Work out the finished part from the listing and answer in its coordinate system (mm). A direction names the side the tool comes from. Round coordinates to 2 decimals unless told otherwise and drop trailing zeros. Write each loop counter-clockwise with the first axis right and the second up, starting at its lowest first coordinate (ties: lowest second). Pieces come first, ordered by that corner, then holes.
1. Flat-ended cylindrical pins translate along their axes: pin 1 Ø1.5 at (x, y) = (16, -24.5) entering from +Z; pin 2 Ø6 at (x, z) = (19, 1) entering from -Y; pin 3 Ø3 at (y, z) = (18.5, 6) entering from -X. Find the tip coordinate at first contact, or state that the pin passes through.
2. Find section B-B (y = 5.5). Write down the section's boundary in (x, z), and give its area (3 significant figures).
3. Find section A-A (x = -22.5). Write down the section's boundary in (y, z), and give its area (3 significant figures).
4. Determine the mould class of faces 1 (the face through (-29, 4, 5)), 2 (the face through (-25.5, 4.3, 4.9)), 3 (the face through (-22, -2.796, 5)) for opening direction X: pulls with the +X half, pulls with the -X half, needs draft (parallel to the pull), parting line crosses it, or undercut.
5. Straight lines are drawn through the part: probe 1 along X at (y, z) = (-19.5, 0.5); probe 2 along Y at (x, z) = (8, 6.5); probe 3 along X at (y, z) = (29, 3.5). For each, find the intervals that lie inside material, in ascending order.
6. A tool of negligible diameter and unlimited length cuts with its end or side. For faces 4 (the face through (-16, -25, 7)), 5 (the face through (22, -2.796, 5)), 6 (the face through (0, 36.204, 7)), 7 (the face through (-17.5, 28, 5)), 8 (the face through (0, 14, 4)), from which of +Z, -Z, +X, -X, +Y, -Y can it reach the whole face along a straight path? Write none if from no direction.
7. Find section C-C (z = 1.25). Count the separate pieces of the cut face and the enclosed holes in it, and give its area (3 significant figures).
```python
from build123d import *

# Parameters (mm, degrees)
F0_W            = 11.5
F0_H            = 14
F1_DEPTH        = 10
F2_W            = 5
F2_H            = 5.5
F2_H_2          = 4
F2_W_2          = 12
F2_H_3          = 5
F3_DEPTH        = 17.501
F7_D            = 5
F8_D            = 6
F9_D            = 6
F9_CSINK_D      = 13.44
F9_CSINK_ANGLE  = 90
F11_D           = 6
F11_CSINK_D     = 13.44
F11_CSINK_ANGLE = 90
F12_R           = 2
F13_R           = 0.99999


# Not quite as in the source:
# - a fillet or chamfer is up to 0.001 mm smaller than in the source, because OpenCascade refuses the exact size


with BuildPart() as f1:
    # F0 (on Top) → F1 (new body)
    with BuildSketch(Plane.XY):
        with Locations((23.25, 4.2037045646)):
            Rectangle(F0_W, F0_H)
        Polygon((17.5, 48.2037045646), (0, 48.2037045646), (0, -25.7962954354), (17.5, -25.7962954354), (17.5, -2.7962954354), (17.5, 11.2037045646), align=None)
    extrude(amount=F1_DEPTH)

    # F2 (on face) → F3 (cut, through all)
    with BuildSketch(Plane.YZ.offset(17.5)):
        Polygon((-25.7962954354, 10), (-25.7962954354, 7), (-11.5389361225, 7), (-8.5389361225, 10), align=None)
        with Locations((-6.2962954354, 2.75)):
            Rectangle(F2_W, F2_H)
        with Locations((13.7037045646, 2)):
            Rectangle(F2_W, F2_H_2)
        with Locations((42.2037045646, 7.5)):
            Rectangle(F2_W_2, F2_H_3)
    extrude(amount=-F3_DEPTH, mode=Mode.SUBTRACT)

    # F7 (through all)
    with Locations(Plane.XY.offset(5)):
        with Locations((10, 41.2037045646)):
            Hole(F7_D / 2)

    # F8 (through all)
    with Locations(Plane.XY.offset(10)):
        with Locations((22.5, 4.2037045646)):
            Hole(F8_D / 2)

    # F9 (through all)
    with Locations(Plane.XY.offset(7)):
        with Locations((11.5, -19.7962954354)):
            CounterSinkHole(F9_D / 2, F9_CSINK_D / 2, counter_sink_angle=F9_CSINK_ANGLE)

    # F11 (through all)
    with Locations(Plane.XY.offset(10)):
        with Locations((10, 28.2037045646)):
            CounterSinkHole(F11_D / 2, F11_CSINK_D / 2, counter_sink_angle=F11_CSINK_ANGLE)

    # F12
    f12_edges = [f1.edges().sort_by_distance(p)[0] for p in [
        (29, -2.796295, 5),
        (29, 11.203705, 5),
        (17.5, 48.203705, 2.5),
        (17.5, -25.796295, 3.5),
    ]]
    fillet(f12_edges, radius=F12_R)

    # F13 (radius 1 in the source; OpenCascade refuses exactly that, so slightly less here)
    f13_edges = [f1.edges().sort_by_distance(p)[0] for p in [
        (17.5, -6.296295, 5.5),
        (8.75, -3.796295, 5.5),
        (8.75, -8.796295, 5.5),
        (17.5, -8.796295, 2.75),
        (17.5, -3.796295, 2.75),
    ]]
    fillet(f13_edges, radius=F13_R)

    # F14: F1 across face


with BuildPart() as f1_1:
    add(f1.part)
    add(f1.part.mirror(Plane(origin=(0, 11.0999568472, 4.6658308471), x_dir=(0, -1, 0), z_dir=(-1, 0, 0))))


solid = f1_1.part
```
Worked answers:
1. pin 1: stops at z = 7
1. pin 2: stops at y = -25.73
1. pin 3: stops at x = -17.5
2. outline: (-29, 0) - (-25.21, 0) - (-25.21, 10) - (-29, 10) - close; (-19.79, 0) - (19.79, 0) - (19.79, 10) - (-19.79, 10) - close; (25.21, 0) - (29, 0) - (29, 10) - (25.21, 10) - close
2. area: 472 mm2
3. outline: (-2.8, 0) - (1.2, 0) - (1.2, 10) - (-2.8, 10) - close; (7.2, 0) - (11.2, 0) - (11.2, 10) - (7.2, 10) - close
3. area: 80.0 mm2
4. face 1: pulls with the -X half
4. face 2: undercut
4. face 3: needs draft
5. probe 1: x = -17.5 to -14.49, -8.51 to 8.51, 14.49 to 17.5
5. probe 2: y = -25.8 to -24.94, -14.65 to 25.68, 30.73 to 36.2
5. probe 3: x = -17.5 to -12.89, -7.11 to 7.11, 12.89 to 17.5
6. face 4: +Z, +X, -X, -Y
6. face 5: +Z, -Z, +X, -Y
6. face 6: +Z, +X, -X, +Y
6. face 7: +Z, -Z, -X, +Y
6. face 8: -Z, +X, -X
7. separate pieces: 3
7. enclosed holes: 8
7. area: 2,350 mm2
